from build123d import *

# Parameters (mm, degrees)
SKETCH1_R           = 32.5
BOSS_EXTRUDE1_DEPTH = 25.4
FILLET1_R           = 6.35
CUT_EXTRUDE1_DEPTH  = 15.621


with BuildPart() as part:
    # Sketch1 → Boss-Extrude1 (new body)
    with BuildSketch(Plane.XY):
        Circle(SKETCH1_R)
    extrude(amount=BOSS_EXTRUDE1_DEPTH)

    # Fillet1
    fillet1_edges = [part.edges().sort_by_distance(p)[0] for p in [
        (-32.5, 0, 0),
        (-32.5, 0, 25.4),
    ]]
    fillet(fillet1_edges, radius=FILLET1_R)

    # Sketch2 → Cut-Extrude1 (cut)
    with BuildSketch(Plane(origin=(0, 0, 0), x_dir=(-1, 0, 0), z_dir=(0, 0, -1))):
        Polygon((3.464101615, -6), (6.92820323, 0), (3.464101615, 6), (-3.464101615, 6), (-6.92820323, 0), (-3.464101615, -6), align=None)
    extrude(amount=-CUT_EXTRUDE1_DEPTH, mode=Mode.SUBTRACT)


solid = part.part
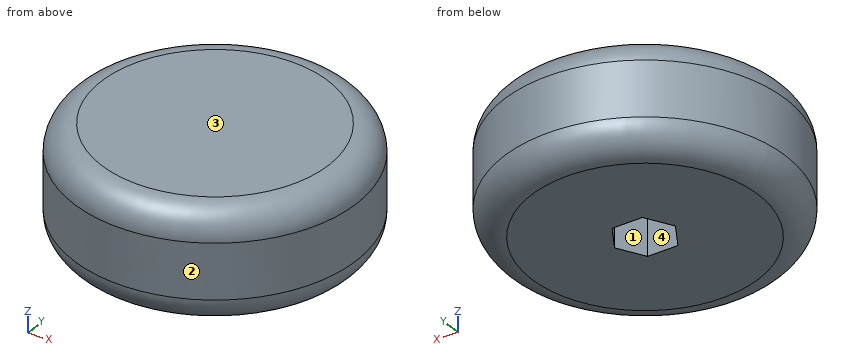
Source: CAD feature listing. Evaluate the final solid. Frame: model axes, mm. Face numbers are marked on the shaded views. Give positions to 0.01 mm unless a question says otherwise; leave off trailing zeros. Loops run counter-clockwise (first coordinate to the right, second up) from the corner with the lowest first, then second, coordinate; pieces in that order, holes last. Notation, with made-up numbers: (-10.75, 11) -> (10.25, 11) arc R5 cw to (10.25, 15) -> close; hole circle Ø4 at (4, 77.25). An arc over 180 degrees is marked (long way). Use a Markdown table: item, result. Add a question column.
1) Pull-direction query (X, two-part tool) for the marked faces 1, 2, 3 and 4; classes: +X half, -X half, draft (parallel to the pull), parting line (faces both ways), or undercut.
2) First-contact query: pin 1 (13 mm diameter, centred on x = 3, y = -3, fed in from -Z); pin 2 (7.5 mm diameter, centred on x = -1, z = 8, fed in from -Y); pin 3 (6 mm diameter, centred on x = -20, z = 16.5, fed in from +Y); pin 4 (1.5 mm diameter, centred on x = 23, y = 23, fed in from +Z). Flat tips, straight axial feed; report the tip coordinate or a pass-through.
3) Line query: line 1 along Y through (x, z) = (-24, 6); line 2 along X through (y, z) = (-2, 14); line 3 along X through (y, z) = (-5.5, 24.5). Output: solid intervals per line, ascending. Write a range as [from, to].
4) Section query B-B, the plane z = 2. Return the cut outline in (x, y).
5) Section query A-A, the plane x = 0. Return the cut outline in (y, z).
Numbers:
| question | item | result |
|---|---|---|
| 1 | face 1 | undercut |
| 1 | face 2 | parting line |
| 1 | face 3 | draft |
| 1 | face 4 | undercut |
| 2 | pin 1 | stops at z = 0 |
| 2 | pin 2 | stops at y = -32.5 |
| 2 | pin 3 | stops at y = 27.7 |
| 2 | pin 4 | stops at z = 21.99 |
| 3 | line 1 | y = [-21.9, 21.9] |
| 3 | line 2 | x = [-32.44, -5.77], [5.77, 32.44] |
| 3 | line 3 | x = [-28.89, 28.89] |
| 4 | outline | circle Ø61.55 at (0, 0); hole (-6.93, 0) -> (-3.46, -6) -> (3.46, -6) -> (6.93, 0) -> (3.46, 6) -> (-3.46, 6) -> close |
| 5 | outline | (-32.5, 6.35) arc R6.35 ccw to (-26.15, 0) -> (-6, 0) -> (-6, 15.62) -> (6, 15.62) -> (6, 0) -> (26.15, 0) arc R6.35 ccw to (32.5, 6.35) -> (32.5, 19.05) arc R6.35 ccw to (26.15, 25.4) -> (-26.15, 25.4) arc R6.35 ccw to (-32.5, 19.05) -> close |
